Source: CAD feature listing. Evaluate the final solid. Frame: model axes, mm. A direction names the side the tool comes from. Coordinates: 2 decimals unless noted, no trailing zeros. Loops run counter-clockwise (first coordinate to the right, second up) from the corner with the lowest first, then second, coordinate; pieces in that order, holes last. Notation, with made-up numbers: M 16,-37.5 L 66,-37.5 A20 cw 66,-6.5 Z; hole C 58.25,28 d2. An arc over 180 degrees is marked long. One line per question, with ' | ' between items. Start each with the question number.
1. Section query D-D, the plane x = 3.5. Output: boundary loops of the cut face in (y, z).
2. Section query C-C, the plane y = -9. Output: boundary loops of the cut face in (x, z).
3. Section query A-A, the plane x = 0. Output: boundary loops of the cut face in (y, z), and give its area (3 significant figures).
4. Access query for faces 1 (the flat face through (2, -7, 2)), 2 (the flat face through (0, 0, 0)), 3 (the flat face through (2, -5, 2)). Directions: +Z, -Z, +X, -X, +Y, -Y. A direction counts if a zero-diameter tool reaches every point of the face in a straight line with its end or side. Return the directions, or none.
5. Section query B-B, the plane z = 0. Output: boundary loops of the cut face in (x, y), and give its area (3 significant figures).
6. Ray query, probe 1 along Y at (x, z) = (-3, -2); probe 2 along X at (y, z) = (-28, -0.25); probe 3 along X at (y, z) = (-33.5, -1.5). Return the intervals inside material, ascending.
7. Pin query (flat end, axial travel): P1, Ø1, axis at x = 1.5, y = -21.5, coming from the -Z side. Return the tip coordinate at first contact, or that it passes through.
```python
from build123d import *

# Parameters (mm, degrees)
F0_R     = 2.5
F1_DEPTH = 5
F2_R     = 4
F3_DEPTH = 2
F4_R     = 2.5
F5_DEPTH = 25
F6_DEPTH = 25


with BuildPart() as f1:
    # F0 (on Front) → F1 (new body)
    with BuildSketch(Plane.XZ):
        Circle(F0_R)
    extrude(amount=F1_DEPTH)

    # F2 (on face) → F3 (join)
    with BuildSketch(Plane.XZ.offset(5)):
        Circle(F2_R)
    extrude(amount=F3_DEPTH)

    # F4 (on face) → F5 (join)
    with BuildSketch(Plane.XZ.offset(7)):
        Circle(F4_R)
    extrude(amount=F5_DEPTH)

    # F6 (add): a face of the model
    f6_faces = [f1.faces().sort_by_distance(p)[0] for p in [
        (0, -32, 0),
    ]]
    extrude(f6_faces, amount=F6_DEPTH)


solid = f1.part
```
Taken from the geometry:
1) outline: M -7,-1.94 L -5,-1.94 L -5,1.94 L -7,1.94 Z
2) outline: C 0,0 d5
3) outline: M -57,-2.5 L -7,-2.5 L -7,-4 L -5,-4 L -5,-2.5 L 0,-2.5 L 0,2.5 L -5,2.5 L -5,4 L -7,4 L -7,2.5 L -57,2.5 Z | area: 291 mm^2
4) face 1: -Y | face 2: +Z, -Z, +X, -X, +Y | face 3: +Y
5) outline: M -4,-7 L -2.5,-7 L -2.5,-57 L 2.5,-57 L 2.5,-7 L 4,-7 L 4,-5 L 2.5,-5 L 2.5,0 L -2.5,0 L -2.5,-5 L -4,-5 Z | area: 291 mm^2
6) probe 1: -7 to -5 | probe 2: -2.49 to 2.49 | probe 3: -2 to 2
7) P1: z = -2.29
